```python
from build123d import *

# Parameters (mm, degrees)
SKETCH1_R           = 2.413
BOSS_EXTRUDE1_DEPTH = 3.175
FILLET1_R           = 10
FILLET2_R           = 2.54
FILLET3_R           = 2.54


with BuildPart() as part:
    # Sketch1 → Boss-Extrude1 (new body)
    with BuildSketch(Plane.XY):
        Polygon((0, 0), (63.5, 0), (108.401280605, 44.901280605), (90.440768363, 62.861792847), (52.978975516, 25.4), (0, 25.4), align=None)
        with Locations((12.7, 12.7)):
            Circle(SKETCH1_R, mode=Mode.SUBTRACT)
        with Locations((31.75, 12.7)):
            Circle(SKETCH1_R, mode=Mode.SUBTRACT)
        with Locations((76.970384182, 31.430896424)):
            Circle(SKETCH1_R, mode=Mode.SUBTRACT)
        with Locations((90.440768363, 44.901280605)):
            Circle(SKETCH1_R, mode=Mode.SUBTRACT)
        with Locations((50.8, 12.7)):
            Circle(SKETCH1_R, mode=Mode.SUBTRACT)
        with Locations((63.5, 17.960512242)):
            Circle(SKETCH1_R, mode=Mode.SUBTRACT)
    extrude(amount=BOSS_EXTRUDE1_DEPTH)

    # Fillet1
    fillet1_edges = [part.edges().sort_by_distance(p)[0] for p in [
        (63.5, 0, 1.5875),
    ]]
    fillet(fillet1_edges, radius=FILLET1_R)

    # Fillet2
    fillet2_edges = [part.edges().sort_by_distance(p)[0] for p in [
        (0, 25.4, 1.5875),
    ]]
    fillet(fillet2_edges, radius=FILLET2_R)

    # Fillet3
    fillet3_edges = [part.edges().sort_by_distance(p)[0] for p in [
        (90.440768363, 62.861792847, 1.5875),
        (108.401280605, 44.901280605, 1.5875),
        (0, 0, 1.5875),
    ]]
    fillet(fillet3_edges, radius=FILLET3_R)


solid = part.part
```
Input: part model. Units: mm. Frame: model coordinates. A direction names the side the tool comes from. Give positions to 0.01 mm unless a question says otherwise; leave off trailing zeros. Order: outer loops, then holes, each group sorted by start corner. A loop starts at its lowest first (then second) coordinate and runs counter-clockwise, first axis right, second up. Notation, with made-up numbers: M 63,-12 L 103,-12 A10 cw 103,1 Z; hole C 8,67 d6. An arc over 180 degrees is marked long. Return JSON: item names as keys, results as strings.
1) Section query B-B on y = 12.7. Output: boundary loops of the cut face in (x, z) (3 decimals), and give its area (3 significant figures).
Taken from the geometry:
{"outline": "M 0,0 L 10.287,0 L 10.287,3.175 L 0,3.175 Z; M 15.113,0 L 29.337,0 L 29.337,3.175 L 15.113,3.175 Z; M 34.163,0 L 48.387,0 L 48.387,3.175 L 34.163,3.175 Z; M 53.213,0 L 76.2,0 L 76.2,3.175 L 53.213,3.175 Z", "area": "196 mm2"}
2) Mould query, pull axis X, two halves, no side actions, for faces 1 (the face through (48.885, 11.232, 1.565)), 2 (the face through (0.724, 24.636, 1.61)), 3 (the face through (107.35, 44.87, 1.61)). Classes: released by +X, released by -X, zero draft, split by the parting line, or undercut.
Taken from the geometry:
{"face 1": "undercut", "face 2": "released by -X", "face 3": "released by +X"}
3) Line query: L1, parallel to Y at x = 50.8, z = 2.15; L2, parallel to Y at x = 6.5, z = 0.85; L3, parallel to X at y = 45.5, z = 1.95. Output: solid intervals per line, ascending. Write a range as [from, to].
Taken from the geometry:
{"L1": "y = [0, 10.29], [15.11, 25.4]", "L2": "y = [0, 25.4]", "L3": "x = [73.08, 88.1], [92.78, 107.28]"}
4) Contact query for flat-ended pins moving along their axis: pin 1 (1.5 mm diameter, centred on x = 58.5, z = 1, fed in from +Y); pin 2 (1.5 mm diameter, centred on y = 30.5, z = 2.5, fed in from +X); pin 3 (1 mm diameter, centred on x = 27.5, z = 2.5, fed in from +Y). Output: stop coordinate, or through.
Taken from the geometry:
{"pin 1": "stops at y = 31.67", "pin 2": "stops at x = 94.75", "pin 3": "stops at y = 25.4"}
5) Section query A-A on x = 50.8. Output: boundary loops of the cut face in (y, z) (3 decimals), and give its area (3 significant figures).
Taken from the geometry:
{"outline": "M 0,0 L 10.287,0 L 10.287,3.175 L 0,3.175 Z; M 15.113,0 L 25.4,0 L 25.4,3.175 L 15.113,3.175 Z", "area": "65.3 mm2"}
6) Access query for faces 4 (the face through (28, 25.4, 2)), 5 (the face through (0.724, 0.764, 1.61)). Directions: +Z, -Z, +X, -X, +Y, -Y. A direction counts if a zero-diameter tool reaches every point of the face in a straight line with its end or side. Return the directions, or none.
Taken from the geometry:
{"face 4": "+Z, -Z, -X, +Y", "face 5": "+Z, -Z, -X, -Y"}
7) Section query C-C on z = 0.7. Output: boundary loops of the cut face in (x, y).
Taken from the geometry:
{"outline": "M 0,2.54 A2.54 ccw 2.54,0 L 59.36,0 A10 ccw 66.43,2.93 L 106.61,43.11 A2.54 ccw 106.61,46.7 L 92.24,61.07 A2.54 ccw 88.64,61.07 L 52.98,25.4 L 2.54,25.4 A2.54 ccw 0,22.86 Z; hole C 12.7,12.7 d4.83; hole C 31.75,12.7 d4.83; hole C 50.8,12.7 d4.83; hole C 63.5,17.96 d4.83; hole C 76.97,31.43 d4.83; hole C 90.44,44.9 d4.83"}
8) Section query D-D on x = 63.5. Output: boundary loops of the cut face in (y, z) (3 decimals), and give its area (3 significant figures).
Taken from the geometry:
{"outline": "M 0.898,0 L 15.548,0 L 15.548,3.175 L 0.898,3.175 Z; M 20.374,0 L 35.921,0 L 35.921,3.175 L 20.374,3.175 Z", "area": "95.9 mm2"}
